Can you work these out from the drawing? Everything is in mm from the part's minimum corner. A direction names the side the tool comes from. Give positions to 0.01 mm unless a question says otherwise; leave off trailing zeros. Order: outer loops, then holes, each group sorted by start corner. A loop starts at its lowest first (then second) coordinate and runs counter-clockwise, first axis right, second up. Notation, with made-up numbers: (37.5, 46.5) - (43.5, 46.5) arc R18 cw to (43.5, 69.5) - close; hole circle Ø1 at (-10, -26). An arc over 180 degrees is marked (long way). Answer as a JSON object with one key per item and string values.
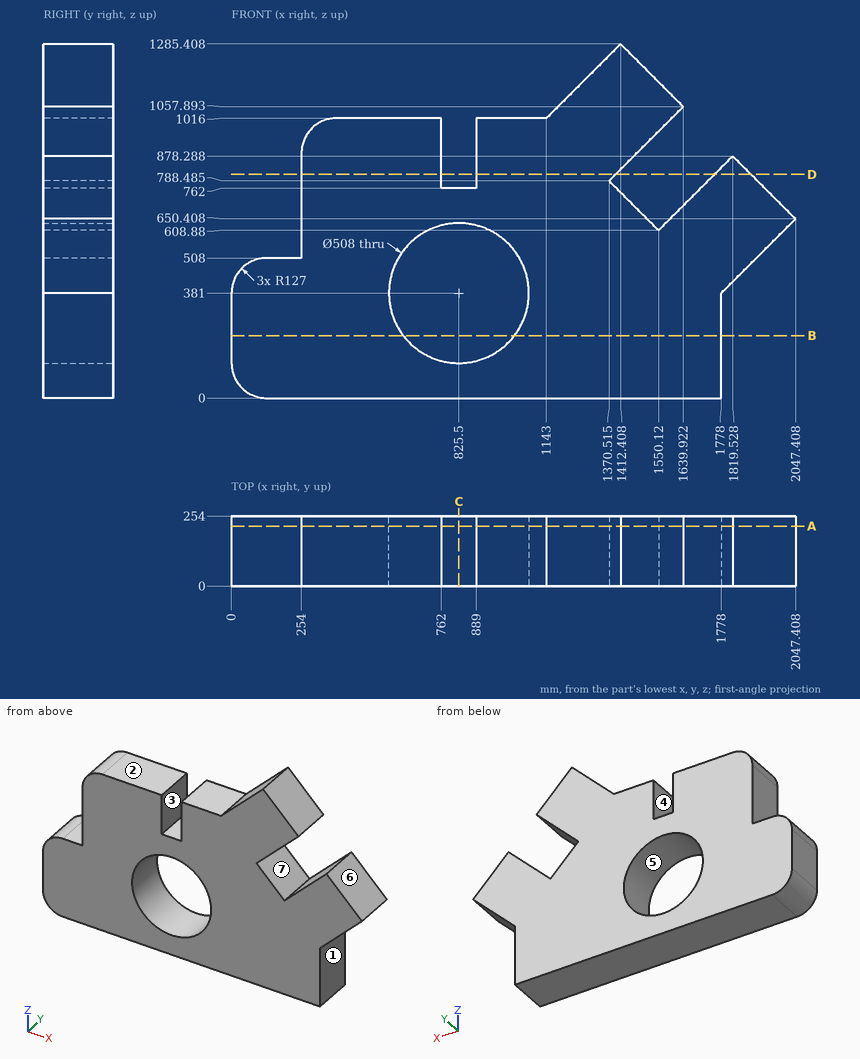
Q1. If we section it at C-C, the plane x = 825.5: Please give me the cut outline in (y, z), then the cut area to 3 significant figures.
Recorded:
{"outline": "(0, 0) - (254, 0) - (254, 127) - (0, 127) - close; (0, 635) - (254, 635) - (254, 762) - (0, 762) - close", "area": "64,500 mm^2"}
Q2. If we section it at B-B, the plane z = 226.5: Please give me the cut outline in (x, y), then the cut area to 3 significant figures.
Recorded:
{"outline": "(0, 0) - (623.89, 0) - (623.89, 254) - (0, 254) - close; (1027.11, 0) - (1778, 0) - (1778, 254) - (1027.11, 254) - close", "area": "349,000 mm^2"}
Q3. We'd pull the mould along Z, two halves only. Please class the marked faces 4, 5, 6 and 7: released by +Z, released by -Z, zero draft, split by the parting line, or undercut.
Recorded:
{"face 4": "zero draft", "face 5": "undercut", "face 6": "released by +Z", "face 7": "undercut"}
Q4. I need wall thicknesses on L1, parallel to X at y = 52, z = 213 (1 decimal); L2, parallel to Z at x = 825, y = 165; L3, parallel to Z at x = 511, y = 80. Which ranges of each line are inside material? Lowest first, please.
Recorded:
{"L1": "x = 0 to 635, 1016 to 1778", "L2": "z = 0 to 127, 635 to 762", "L3": "z = 0 to 1016"}
Q5. If we section it at D-D, the plane z = 812.5: Please give me the cut outline in (x, y) (1 decimal), then the cut area to 3 significant figures.
Recorded:
{"outline": "(254, 0) - (762, 0) - (762, 254) - (254, 254) - close; (889, 0) - (1394.5, 0) - (1394.5, 254) - (889, 254) - close; (1753.7, 0) - (1885.3, 0) - (1885.3, 254) - (1753.7, 254) - close", "area": "291,000 mm^2"}
Q6. Which directions (+Z, -Z, +X, -X, +Y, -Y) give clear straight access to the entire face, cutting with the end or side of a thin tool? Please do the marked faces 1, 2 and 3.
Recorded:
{"face 1": "-Z, +X, +Y, -Y", "face 2": "+Z, -X, +Y, -Y", "face 3": "+Z, +Y, -Y"}
Q7. If we section it at A-A, the plane y = 217.5: Please give me the cut outline in (x, z) (1 decimal).
Recorded:
{"outline": "(0, 127) arc R127 ccw to (127, 0) - (1778, 0) - (1778, 381) - (2047.4, 650.4) - (1819.5, 878.3) - (1550.1, 608.9) - (1370.5, 788.5) - (1639.9, 1057.9) - (1412.4, 1285.4) - (1143, 1016) - (889, 1016) - (889, 762) - (762, 762) - (762, 1016) - (381, 1016) arc R127 ccw to (254, 889) - (254, 508) - (127, 508) arc R127 ccw to (0, 381) - close; hole circle Ø508 at (825.5, 381)"}
Q8. I'm going to push flat-ended pins straight in: pin 1 Ø1.5 at (y, z) = (137.5, 1015) entering from +X; pin 2 Ø1 at (y, z) = (141.5, 179) entering from +X; pin 3 Ø2 at (y, z) = (159.5, 521.5) entering from -X. Where does each tip first touch, or does it pass through?
Recorded:
{"pin 1": "stops at x = 1597.78", "pin 2": "stops at x = 1778", "pin 3": "stops at x = 254"}
